For this review, take the finished solid that the model builds, in its own axes (mm). Face numbers are marked on the shaded views. A direction names the side the tool comes from. Give positions to 0.01 mm unless a question says otherwise; leave off trailing zeros. Order: outer loops, then holes, each group sorted by start corner. A loop starts at its lowest first (then second) coordinate and runs counter-clockwise, first axis right, second up. Notation, with made-up numbers: (20, 83) -> (50, 83) arc R22 cw to (50, 107) -> close; hole circle Ø4 at (42, -11). An arc over 180 degrees is marked (long way). Return JSON: item names as keys, results as strings. Group by question number.
1) Add section C-C (y = 441). Give the boundary of the cut face in (x, z), then the cut area to 3 significant figures.
2) Insertion check: P1, Ø6, axis at y = 757, z = 12, coming from the -X side; P2, Ø10, axis at y = 624, z = 15.5, coming from the -X side. Each pin has a flat end and moves straight along its axis. Give the tip position at first contact, or say it passes through.
3) Add section D-D (x = 0). Give the boundary of the cut face in (y, z).
4) Add section A-A (z = 0). Give the boundary of the cut face in (x, y).
5) To check wall thickness, follow line 1 along X through (y, z) = (366.5, -4.5); line 2 along X through (y, z) = (943, 2.5); line 3 along Z through (x, y) = (0, 570). State the ranges of each line that lie inside material, in increasing order.
6) For the marked faces 1, 2 and 3, list the 3-axis set-ups (+Z, -Z, +X, -X, +Y, -Y) from which the entire face can be reached by the end or side of a thin tool; tool diameter is ignored.
7) Add section B-B (x = 743.5). Give the boundary of the cut face in (y, z).
from build123d import *

# Parameters (mm, degrees)
SKETCH1_W           = 10
SKETCH1_H           = 1260
SKETCH2_W           = 1115
SKETCH2_H           = 1260
SKETCH2_W_2         = 915
SKETCH2_H_2         = 1060
BOSS_EXTRUDE1_DEPTH = 25
SKETCH3_W           = 50
SKETCH3_H           = 1260
BOSS_EXTRUDE2_DEPTH = 10


with BuildPart() as part:
    # Sketch1 → Revolve1 (revolve)
    with BuildSketch(Plane.XY):
        with Locations((-55, 630)):
            Rectangle(SKETCH1_W, SKETCH1_H)
    revolve(axis=Axis((0, 0, 0), (0, 1, 0)))



with BuildPart() as body_2:
    # Sketch2 → Boss-Extrude1 (new body, symmetric)
    with BuildSketch(Plane.XY):
        with Locations((617.5, 630)):
            Rectangle(SKETCH2_W, SKETCH2_H)
        with Locations((617.5, 630)):
            Rectangle(SKETCH2_W_2, SKETCH2_H_2, mode=Mode.SUBTRACT)
    extrude(amount=BOSS_EXTRUDE1_DEPTH, both=True)


with BuildPart() as part_1:
    add(part.part)

    add(body_2.part)  # Boss-Extrude2 merges body 2
    # Sketch3 → Boss-Extrude2 (add)
    with BuildSketch(Plane.ZY.offset(-60)):
        with Locations((0, 630)):
            Rectangle(SKETCH3_W, SKETCH3_H)
    extrude(amount=BOSS_EXTRUDE2_DEPTH)


solid = part_1.part
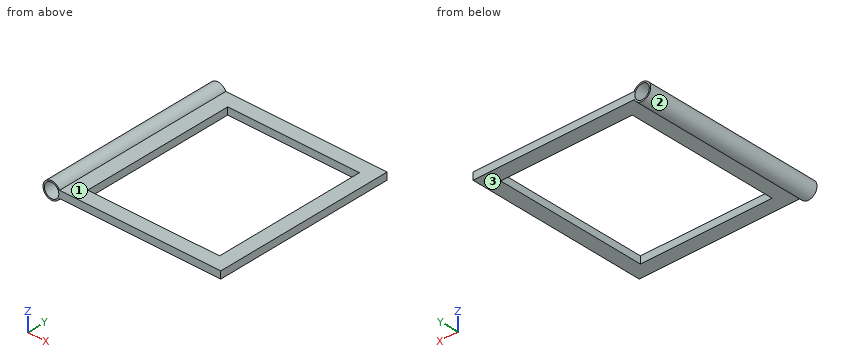
Evaluation:
{
 "1": {"outline": "(54.54, -25) -> (160, -25) -> (160, 25) -> (54.54, 25) arc R60 ccw (long way) to start; (1075, -25) -> (1175, -25) -> (1175, 25) -> (1075, 25) -> close; hole circle Ø100 at (0, 0)", "area": "13,500 mm^2"},
 "2": {"P1": "x = -59.32", "P2": "x = -59.07"},
 "3": {"outline": "(0, -60) -> (1260, -60) -> (1260, -50) -> (0, -50) -> close; (0, 50) -> (1260, 50) -> (1260, 60) -> (0, 60) -> close"},
 "4": {"outline": "(-60, 0) -> (-50, 0) -> (-50, 1260) -> (-60, 1260) -> close; (50, 0) -> (1175, 0) -> (1175, 1260) -> (50, 1260) -> close; hole (160, 100) -> (1075, 100) -> (1075, 1160) -> (160, 1160) -> close"},
 "5": {"line 1": "-59.83 to -49.8, 49.8 to 160, 1075 to 1175", "line 2": "-59.95 to -49.94, 49.94 to 160, 1075 to 1175", "line 3": "-60 to -50, 50 to 60"},
 "6": {"face 1": "+Z, +X, +Y, -Y", "face 2": "+Y, -Y", "face 3": "-Z, +X, +Y, -Y"},
 "7": {"outline": "(0, -25) -> (100, -25) -> (100, 25) -> (0, 25) -> close; (1160, -25) -> (1260, -25) -> (1260, 25) -> (1160, 25) -> close"}
}
